Model file for the job. Use its own axes, mm. A direction names the side the tool comes from. Round coordinates to 2 decimals unless told otherwise and drop trailing zeros. Order: outer loops, then holes, each group sorted by start corner. A loop starts at its lowest first (then second) coordinate and runs counter-clockwise, first axis right, second up. Notation, with made-up numbers: (-12.5, 20) -> (46.5, 20) arc R28 cw to (46.5, 49) -> close; hole circle Ø8 at (19, 50). An arc over 180 degrees is marked (long way). Put each result on its own line as item: value. Start each with the question number.
Q1. 3-axis set-ups, long thin cutter, end or side, ignore diameter. For faces 4 (the face through (134.49, 1.08, 67.15)), 5 (the face through (246.863, 1.085, 141.692)): which of +Z, -Z, +X, -X, +Y, -Y reach the whole face in a straight line?
Q2. Probe L1, parallel to X at y = 1.5, z = -20.5; L2, parallel to X at y = 0.95, z = -141; L3, parallel to X at y = 0.4, z = -40.5. List the from-to ranges inside material, lowest first.
Q3. Cut at B-B, the plane y = 0.6. State how many separate pieces and enclosed holes the cut face has, and give its area (3 significant figures).
Q4. Pull direction Z, two halves, no side cores. Call faces 1 (the face through (99, 0, -2)), 2 (the face through (134.65, 1.08, -66.99)), 3 (the face through (246.692, 1.085, -141.863)): released by +Z, released by -Z, zero draft, split by the parting line, or undercut.
Q5. Cut at A-A, the plane z = 42.5. List the corners of the cut face in (x, y).
from build123d import *

# Parameters (mm, degrees)
SKETCH1_R           = 1.6
SKETCH1_R_2         = 1.4
SKETCH1_W           = 10
SKETCH1_H           = 34
BOSS_EXTRUDE1_DEPTH = 2.2
SKETCH2_R           = 1.35
CUT_EXTRUDE1_DEPTH  = 59.2
SKETCH4_W           = 292.714783979
SKETCH4_H           = 326.007375252
CUT_EXTRUDE2_DEPTH  = 2.2


with BuildPart() as part:
    # Sketch1 → Boss-Extrude1 (new body)
    with BuildSketch(Plane(origin=(0, 0, 0), x_dir=(1, 0, 0), z_dir=(0, 1, 0))):
        with BuildLine():
            Line((-239, 145), (239, 145))
            ThreePointArc((239, 145), (246.778174593, 141.778174593), (250, 134))
            Line((250, 134), (250, -134))
            ThreePointArc((250, -134), (246.778174593, -141.778174593), (239, -145))
            Line((239, -145), (-239, -145))
            ThreePointArc((-239, -145), (-246.778174593, -141.778174593), (-250, -134))
            Line((-250, -134), (-250, 134))
            ThreePointArc((-250, 134), (-246.778174593, 141.778174593), (-239, 145))
        make_face()
        with Locations(Location((63.75, 141, 0), (0, 0, 270))):
            Circle(SKETCH1_R, mode=Mode.SUBTRACT)
        with Locations(Location((184.75, 141, 0), (0, 0, 270))):
            Circle(SKETCH1_R, mode=Mode.SUBTRACT)
        with Locations(Location((246, 68.5, 0), (0, 0, 270))):
            Circle(SKETCH1_R, mode=Mode.SUBTRACT)
        with Locations(Location((0, 103.5, 0), (0, 0, 270))):
            Circle(SKETCH1_R_2, mode=Mode.SUBTRACT)
        with Locations(Location((0, -103.5, 0), (0, 0, 270))):
            Circle(SKETCH1_R_2, mode=Mode.SUBTRACT)
        with Locations(Location((-246, 68.5, 0), (0, 0, 90))):
            Circle(SKETCH1_R, mode=Mode.SUBTRACT)
        with Locations(Location((-184.75, 141, 0), (0, 0, 90))):
            Circle(SKETCH1_R, mode=Mode.SUBTRACT)
        with Locations(Location((-63.75, 141, 0), (0, 0, 90))):
            Circle(SKETCH1_R, mode=Mode.SUBTRACT)
        with Locations(Location((184.75, -141, 0), (0, 0, 90))):
            Circle(SKETCH1_R, mode=Mode.SUBTRACT)
        with Locations(Location((246, -68.5, 0), (0, 0, 90))):
            Circle(SKETCH1_R, mode=Mode.SUBTRACT)
        with Locations(Location((63.75, -141, 0), (0, 0, 90))):
            Circle(SKETCH1_R, mode=Mode.SUBTRACT)
        with Locations(Location((-63.75, -141, 0), (0, 0, 270))):
            Circle(SKETCH1_R, mode=Mode.SUBTRACT)
        with Locations(Location((-184.75, -141, 0), (0, 0, 270))):
            Circle(SKETCH1_R, mode=Mode.SUBTRACT)
        with Locations(Location((-246, -68.5, 0), (0, 0, 270))):
            Circle(SKETCH1_R, mode=Mode.SUBTRACT)
        with BuildLine():
            Line((-127.5, -70), (-122.5, -70))
            ThreePointArc((-122.5, -70), (-115.428932188, -67.071067812), (-112.5, -60))
            Line((-112.5, -60), (-112.5, 60))
            ThreePointArc((-112.5, 60), (-115.428932188, 67.071067812), (-122.5, 70))
            Line((-122.5, 70), (-127.5, 70))
            ThreePointArc((-127.5, 70), (-134.571067812, 67.071067812), (-137.5, 60))
            Line((-137.5, 60), (-137.5, -60))
            ThreePointArc((-137.5, -60), (-134.571067812, -67.071067812), (-127.5, -70))
        make_face(mode=Mode.SUBTRACT)
        with BuildLine():
            Line((122.5, -70), (127.5, -70))
            ThreePointArc((127.5, -70), (134.571067812, -67.071067812), (137.5, -60))
            Line((137.5, -60), (137.5, 60))
            ThreePointArc((137.5, 60), (134.571067812, 67.071067812), (127.5, 70))
            Line((127.5, 70), (122.5, 70))
            ThreePointArc((122.5, 70), (115.428932188, 67.071067812), (112.5, 60))
            Line((112.5, 60), (112.5, -60))
            ThreePointArc((112.5, -60), (115.428932188, -67.071067812), (122.5, -70))
        make_face(mode=Mode.SUBTRACT)
        with Locations((0, 45)):
            Rectangle(SKETCH1_W, SKETCH1_H, mode=Mode.SUBTRACT)
    extrude(amount=BOSS_EXTRUDE1_DEPTH)

    # Sketch2 → Cut-Extrude1 (cut)
    with BuildSketch(Plane(origin=(0, 2.2, 0), x_dir=(1, 0, 0), z_dir=(0, 1, 0))):
        with Locations(Location((-6, -18.5, 0), (0, 0, 270))):
            Circle(SKETCH2_R)
        with Locations(Location((6, -18.5, 0), (0, 0, 270))):
            Circle(SKETCH2_R)
        with Locations(Location((-6, -98.5, 0), (0, 0, 270))):
            Circle(SKETCH2_R)
        with Locations(Location((6, -98.5, 0), (0, 0, 270))):
            Circle(SKETCH2_R)
        with Locations(Location((-6, 123.5, 0), (0, 0, 270))):
            Circle(SKETCH2_R)
        with Locations(Location((6, 123.5, 0), (0, 0, 270))):
            Circle(SKETCH2_R)
        with Locations(Location((-6, 83.5, 0), (0, 0, 270))):
            Circle(SKETCH2_R)
        with Locations(Location((6, 83.5, 0), (0, 0, 270))):
            Circle(SKETCH2_R)
    extrude(amount=-CUT_EXTRUDE1_DEPTH, mode=Mode.SUBTRACT)

    # Sketch4 → Cut-Extrude2 (cut)
    with BuildSketch(Plane(origin=(0, 2.2, 0), x_dir=(1, 0, 0), z_dir=(0, 1, 0))):
        with Locations((-146.35739199, -18.003687626)):
            Rectangle(SKETCH4_W, SKETCH4_H)
    extrude(amount=-CUT_EXTRUDE2_DEPTH, mode=Mode.SUBTRACT)


solid = part.part
Ans:
1. face 4: +Y, -Y
1. face 5: +Z, +X, +Y, -Y
2. L1: x = 0 to 112.5, 137.5 to 250
2. L2: x = 0 to 62.15, 65.35 to 183.15, 186.35 to 247.49
2. L3: x = 5 to 112.5, 137.5 to 250
3. separate pieces: 1
3. enclosed holes: 11
3. area: 68,800 mm^2
4. face 1: zero draft
4. face 2: undercut
4. face 3: released by -Z
5. outline: (0, 0) -> (112.5, 0) -> (112.5, 2.2) -> (0, 2.2) -> close; (137.5, 0) -> (250, 0) -> (250, 2.2) -> (137.5, 2.2) -> close
